from build123d import *

# Parameters (mm, degrees)
BOSS_EXTRUDE1_DEPTH          = 9.525
F_1_8_0_125_DIAMETER_HOLE1_D = 3.175


with BuildPart() as part:
    # Sketch1 → Boss-Extrude1 (new body)
    with BuildSketch(Plane(origin=(0, 0, 0), x_dir=(1, 0, 0), z_dir=(0, 1, 0))):
        Polygon((0, 0), (12.7, 0), (12.7, -9.525), (11.1125, -9.525), (11.1125, -1.5875), (0, -1.5875), align=None)
    extrude(amount=BOSS_EXTRUDE1_DEPTH)

    # 1/8 (0.125) Diameter Hole1 (through all)
    with Locations(Plane.ZY.offset(-11.1125)):
        with Locations((6.35, 4.7625)):
            Hole(F_1_8_0_125_DIAMETER_HOLE1_D / 2)


solid = part.part
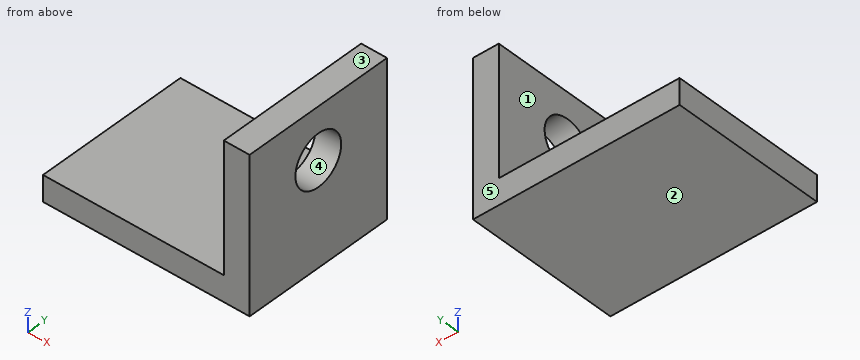
Can you work these out from the model? Positions are in its coordinate system, mm. Face numbers are marked on the shaded views. A direction names the side the tool comes from. Round coordinates to 2 decimals unless told otherwise and drop trailing zeros. Loops run counter-clockwise (first coordinate to the right, second up) from the corner with the lowest first, then second, coordinate; pieces in that order, holes last. Notation, with made-up numbers: (50.25, -29) - (96.25, -29) arc R16 ccw to (96.25, -11) - close; hole circle Ø7 at (83.5, 57). An arc over 180 degrees is marked (long way). Answer in a Markdown table with one row per item. Add a question column.
Q1. I need wall thicknesses on L1, parallel to Y at x = 12.2, z = 6.35 (3 decimals); L2, parallel to Z at x = 2.25, y = 8; L3, parallel to X at y = 5.75, z = 4. Which ranges of each line are inside material? Lowest first, please.
Q2. Which directions (+Z, -Z, +X, -X, +Y, -Y) give clear straight access to the entire face, cutting with the end or side of a thin tool? Please do the marked faces 1 and 2.
Q3. I want a section at B-B on y = 5.25. List the corners of the cut face in (x, z) for me (1 decimal), and give its area (3 significant figures).
Q4. I want a section at D-D on z = 8.25. List the corners of the cut face in (x, y) for me (1 decimal).
Q5. I want a section at C-C on y = 3. List the corners of the cut face in (x, z) for me (1 decimal).
Q6. For pin 1 Ø2.5 at (y, z) = (6, 5.5) entering from -X, with a flat end and sliding along its axis, tell me the tip position at first contact or that it passes through.
Q7. We'd pull the mould along Z, two halves only. Please class the marked faces 3, 4 and 5: pulls with the +Z half, pulls with the -Z half, needs draft (parallel to the pull), parting line crosses it, or undercut.
A:
| question | item | result |
|---|---|---|
| 1 | L1 | 0 to 3.175, 6.35 to 9.525 |
| 1 | L2 | 0 to 1.59 |
| 1 | L3 | 11.11 to 12.7 |
| 2 | face 1 | +Z, -X, +Y, -Y |
| 2 | face 2 | -Z, +X, -X, +Y, -Y |
| 3 | outline | (0, 0) - (12.7, 0) - (12.7, 4.8) - (11.1, 4.8) - (11.1, 1.6) - (0, 1.6) - close; (11.1, 7.9) - (12.7, 7.9) - (12.7, 9.5) - (11.1, 9.5) - close |
| 3 | area | 28.0 mm^2 |
| 4 | outline | (11.1, 0) - (12.7, 0) - (12.7, 9.5) - (11.1, 9.5) - close |
| 5 | outline | (0, 0) - (12.7, 0) - (12.7, 9.5) - (11.1, 9.5) - (11.1, 1.6) - (0, 1.6) - close |
| 6 | pin 1 | x = 11.11 |
| 7 | face 3 | pulls with the +Z half |
| 7 | face 4 | undercut |
| 7 | face 5 | needs draft |
